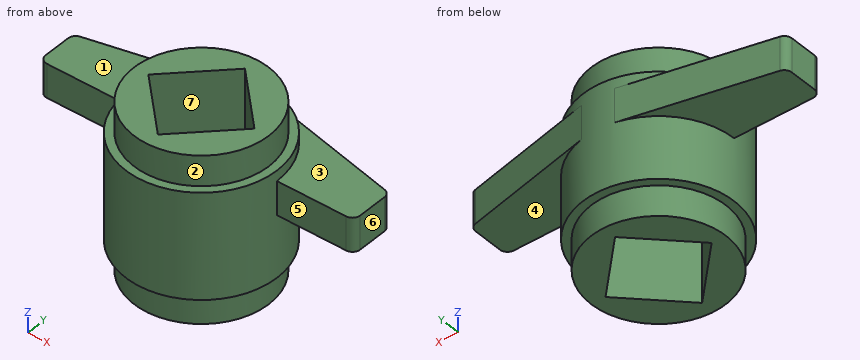
from build123d import *

# Parameters (mm, degrees)
F0_R      = 7.85
F1_DEPTH  = 11
F2_R      = 7
F3_DEPTH  = 3.13
F4_R      = 7
F5_DEPTH  = 3.13
F7_DEPTH  = 17.261
F10_DEPTH = 3.5


with BuildPart() as f1:
    # F0 (on Top) → F1 (new body)
    with BuildSketch(Plane.XY):
        Circle(F0_R)
    extrude(amount=F1_DEPTH)

    # F2 (on face) → F3 (join)
    with BuildSketch(Plane.XY.offset(11)):
        Circle(F2_R)
    extrude(amount=F3_DEPTH)

    # F4 (on face) → F5 (join)
    with BuildSketch(Plane(origin=(0, 0, 0), x_dir=(1, 0, 0), z_dir=(0, 0, -1))):
        Circle(F4_R)
    extrude(amount=F5_DEPTH)

    # F6 (on face) → F7 (cut, through all)
    with BuildSketch(Plane.XY.offset(14.13)):
        Polygon((5.5154328933, 0), (0, 5.5154328933), (0, 0), align=None)
        Polygon((0, 0), (0, 5.5154328933), (-5.5154328933, 0), align=None)
        Polygon((5.5154328933, 0), (0, 0), (0, -5.5154328933), align=None)
        Polygon((0, -5.5154328933), (0, 0), (-5.5154328933, 0), align=None)
    extrude(amount=-F7_DEPTH, mode=Mode.SUBTRACT)

    # F9 (on offset) → F10 (join)
    with BuildSketch(Plane.XY.offset(9.93)):
        with BuildLine():
            Line((-16.05, 0), (-7.85, 0))
            ThreePointArc((-7.85, 0), (-6.1265149302, 4.9079848013), (-1.7128497301, 7.6608515063))
            Line((-1.7128497301, 7.6608515063), (-16.2245579343, 4.41625455))
            ThreePointArc((-16.2245579343, 4.41625455), (-16.6743582095, 4.1357076247), (-16.85, 3.6355308296))
            Line((-16.85, 3.6355308296), (-16.85, 0.8))
            ThreePointArc((-16.85, 0.8), (-16.6156854249, 0.2343145751), (-16.05, 0))
        make_face()
        with BuildLine():
            ThreePointArc((1.7128497301, 7.6608515063), (6.1265149302, 4.9079848013), (7.85, 0))
            Line((7.85, 0), (15.05, 0))
            ThreePointArc((15.05, 0), (15.6156854249, 0.2343145751), (15.85, 0.8))
            Line((15.85, 0.8), (15.85, 3.8591156007))
            ThreePointArc((15.85, 3.8591156007), (15.6743582095, 4.3592923957), (15.2245579343, 4.6398393211))
            Line((15.2245579343, 4.6398393211), (1.7128497301, 7.6608515063))
        make_face()
    extrude(amount=-F10_DEPTH)


solid = f1.part
Read the model definition and answer for the solid it produces. Units are mm, in the model's axes. Face numbers are marked on the shaded views. A direction names the side the tool comes from. Coordinates: 2 decimals unless noted, no trailing zeros. Order: outer loops, then holes, each group sorted by start corner. A loop starts at its lowest first (then second) coordinate and runs counter-clockwise, first axis right, second up. Notation, with made-up numbers: (-16.5, 84.5) - (21.5, 84.5) arc R28 cw to (21.5, 105.5) - close; hole circle Ø6 at (4.5, 82). An arc over 180 degrees is marked (long way). Use one line per item in the form item = value.
(1) Section A-A, the plane z = 7.25 is taken. Give the vertices of the cut face in (x, y), then the cut area to 3 significant figures.
Computed values:
outline = (-16.85, 0.8) arc R0.8 ccw to (-16.05, 0) - (-7.85, 0) arc R7.85 ccw to (7.85, 0) - (15.05, 0) arc R0.8 ccw to (15.85, 0.8) - (15.85, 3.86) arc R0.8 ccw to (15.22, 4.64) - (1.71, 7.66) arc R7.85 ccw to (-1.71, 7.66) - (-16.22, 4.42) arc R0.8 ccw to (-16.85, 3.64) - close; hole (-5.52, 0) - (0, -5.52) - (5.52, 0) - (0, 5.52) - close
area = 239 mm²
(2) Section D-D, the plane z = -0.5 is taken. Give the vertices of the cut face in (x, y).
Computed values:
outline = circle Ø14 at (0, 0); hole (-5.52, 0) - (0, -5.52) - (5.52, 0) - (0, 5.52) - close
(3) Which of the six approach directions +Z, -Z, +X, -X, +Y, -Y give full straight-line access (tool end or side, diameter ignored) to the marked faces 1, 2, 3 and 4?
Computed values:
face_1 = +Z, -X, +Y
face_2 = +Z
face_3 = +Z, +X, +Y
face_4 = -Z, +X, +Y
(4) Section B-B, the plane y = -3 is taken. Give the vertices of the cut face in (x, z), then the cut area to 3 significant figures.
Computed values:
outline = (-7.25, 0) - (-6.32, 0) - (-6.32, -3.13) - (-2.52, -3.13) - (-2.52, 14.13) - (-6.32, 14.13) - (-6.32, 11) - (-7.25, 11) - close; (2.52, -3.13) - (6.32, -3.13) - (6.32, 0) - (7.25, 0) - (7.25, 11) - (6.32, 11) - (6.32, 14.13) - (2.52, 14.13) - close
area = 152 mm²
(5) Given pin 1 Ø2.5 at (x, y) = (-10.5, 4) entering from +Z; pin 2 Ø5 at (y, z) = (-2, 6) entering from -X; pin 3 Ø3 at (x, z) = (11.5, 8) entering from -Y; pin 4 Ø8 at (x, z) = (-4, 9.5) entering from -Y, each flat-ended and moving along its own axis, determine where each tip first touches the part or whether it passes through.
Computed values:
pin_1 = 9.93
pin_2 = -16.78
pin_3 = 0
pin_4 = -7.85
(6) Section C-C, the plane x = -5 is taken. Give the vertices of the cut face in (y, z).
Computed values:
outline = (-6.05, 0) - (-4.9, 0) - (-4.9, -3.13) - (-0.52, -3.13) - (-0.52, 14.13) - (-4.9, 14.13) - (-4.9, 11) - (-6.05, 11) - close; (0.52, -3.13) - (4.9, -3.13) - (4.9, 0) - (6.05, 0) - (6.05, 6.43) - (6.93, 6.43) - (6.93, 9.93) - (6.05, 9.93) - (6.05, 11) - (4.9, 11) - (4.9, 14.13) - (0.52, 14.13) - close
(7) For a pull along X with two mould halves and no side action, classify the marked faces 5, 6 and 7 as pulls with the +X half, pulls with the -X half, needs draft (parallel to the pull), parting line crosses it, or undercut.
Computed values:
face_5 = needs draft
face_6 = pulls with the +X half
face_7 = undercut
(8) Straight lines are drawn through the part: L1, parallel to Z at x = -1, y = -7; L2, parallel to X at y = -3, z = 5.75. For each, find the intervals that lie inside material, in ascending order.
Computed values:
L1 = 0 to 11
L2 = -7.25 to -2.52, 2.52 to 7.25
